The model under review builds one solid part; all positions refer to its coordinate system, in mm. A direction names the side the tool comes from. Coordinates: 2 decimals unless noted, no trailing zeros. Loops run counter-clockwise (first coordinate to the right, second up) from the corner with the lowest first, then second, coordinate; pieces in that order, holes last. Notation, with made-up numbers: M -19.5,45.5 L 16.5,45.5 A16 ccw 16.5,74.5 Z; hole C 14.25,42.5 d7. An arc over 180 degrees is marked long. One line per item, written item: value.
```python
from build123d import *

# Parameters (mm, degrees)
F0_W          = 41.3257516921
F0_H          = 115.0570958853
F1_DEPTH      = 8
F3_DEPTH      = 16
F5_DEPTH      = 8.5
F6_R          = 4
F7_R          = 10
F9_D          = 5
F10_R         = 1
F12_DEPTH     = 8
F13_T4_ANGLE  = 50.4345634546
F13_S5_R      = 29.5691559209
F13_T6_DEPTH  = 16
F13_T11_ANGLE = 49.9258142249
F13_S12_R     = 29.5691559209
F13_T13_DEPTH = 16
F14_W         = 7.5
F14_H         = 18
F15_DEPTH     = 3
F16_R         = 1


# Not quite as in the source:
# - a fillet or chamfer that OpenCascade refuses, or shapes differently, is made with other operations: its cross-section is extruded or revolved along the edge and cut away or added
# - a pattern or mirror of a feature is missing from the dataset's text; its kind, count and spacing are read off the source's solid


with BuildPart() as f1:
    # F0 (on Front) → F1 (new body)
    with BuildSketch(Plane.XZ):
        Rectangle(F0_W, F0_H)
    extrude(amount=F1_DEPTH)

    # F2 (on face) → F3 (join)
    with BuildSketch(Plane.XZ):
        with BuildLine():
            Line((20.662875846, -21.1513721457), (20.662875846, 21.1513721457))
            ThreePointArc((20.662875846, 21.1513721457), (0, 29.5691559209), (-20.662875846, 21.1513721457))
            Line((-20.662875846, 21.1513721457), (-20.662875846, -21.1513721457))
            ThreePointArc((-20.662875846, -21.1513721457), (0, -29.5691559209), (20.662875846, -21.1513721457))
        make_face()
        with BuildLine():
            ThreePointArc((20.662875846, -21.1513721457), (27.251777736, -11.4749985666), (29.5691559209, 0))
            ThreePointArc((29.5691559209, 0), (27.251777736, 11.4749985666), (20.662875846, 21.1513721457))
            Line((20.662875846, 21.1513721457), (20.662875846, -21.1513721457))
        make_face()
    extrude(amount=F3_DEPTH)

    # F4 (on face) → F5 (cut)
    with BuildSketch(Plane(origin=(0, 0, 0), x_dir=(-1, 0, 0), z_dir=(0, 1, 0))):
        Polygon((5.0357980654, 39.4895523787), (5.0357980654, 47.5048683584), (-5.0371875986, 47.5048683584), (-5.0371875986, 39.4847430289), align=None)
    f5 = extrude(amount=-F5_DEPTH, mode=Mode.SUBTRACT)

    # F5_copies: F5 across plane
    add(f5.mirror(Plane(origin=(0, 0, 0), x_dir=(-1, 0, 0), z_dir=(0, 0, -1))), mode=Mode.SUBTRACT)

    # F6
    f6_edges = [f1.edges().sort_by_distance(p)[0] for p in [
        (5.037188, -4, -47.504868),
        (-5.035798, -4, -47.504868),
        (5.037188, -4, -39.484743),
        (-5.035798, -4, -39.489552),
        (-5.035798, -4, 47.504868),
        (-5.035798, -4, 39.489552),
        (5.037188, -4, 39.484743),
        (5.037188, -4, 47.504868),
    ]]
    fillet(f6_edges, radius=F6_R)

    # F7
    f7_edges = [f1.edges().sort_by_distance(p)[0] for p in [
        (20.662876, -4, 57.528548),
        (-20.662876, -4, 57.528548),
        (-20.662876, -4, -57.528548),
        (20.662876, -4, -57.528548),
    ]]
    fillet(f7_edges, radius=F7_R)

    # F8: union 

    # F9 (through all)
    with Locations(Plane(origin=(0, 0, 0), x_dir=(1, 0, 0), z_dir=(0, 1, 0))):
        with Locations((22.990738973, 0), (-11.4866392687, -19.9111644179), (-11.4866392687, 19.9130717665)):
            Hole(F9_D / 2)

    # F10
    f10_edges = [f1.edges().sort_by_distance(p)[0] for p in [
        (-20.662876, -8, 34.33996),
        (-20.662876, -8, -34.33996),
    ]]
    fillet(f10_edges, radius=F10_R)

    # F11 (on face) → F12 (join)
    with BuildSketch(Plane.XZ.offset(16)):
        with BuildLine():
            ThreePointArc((-20.662875846, 21.1513721457), (-27.2355425635, 11.47094423), (-29.5438040048, 0))
            ThreePointArc((-29.5438040048, 0), (-27.2133537023, -11.4616276864), (-20.662875846, -21.1513721457))
            Line((-20.662875846, -21.1513721457), (-20.662875846, 21.1513721457))
        make_face()
    extrude(amount=-F12_DEPTH)

    # F13: fillet of radius 1 on 2 edges, made by hand


with BuildPart() as f13_tool2:
    # F13_s3 → F13_t4 (revolve)
    with BuildSketch(Plane(origin=(0.039948819, 0, 0.0330329638), x_dir=(0, 1, 0), z_dir=(0.7706607763, 0, 0.6372456103))):
        with BuildLine():
            ThreePointArc((-9, 29.573386115), (-8.2928932188, 29.2804928962), (-8, 28.573386115))
            Line((-8, 28.573386115), (-7.98, 28.573386115))
            Line((-7.98, 28.573386115), (-7.98, 29.593386115))
            Line((-7.98, 29.593386115), (-9, 29.593386115))
            Line((-9, 29.593386115), (-9, 29.573386115))
        make_face()
    revolve(axis=Axis((0.058163466, -8, 0.0110048576), (0, -1, 0)), revolution_arc=F13_T4_ANGLE)

    # F13_s5 → F13_t6 (intersect, symmetric)
    with BuildSketch(Plane.XZ.offset(8.5)):
        Circle(F13_S5_R)
    extrude(amount=F13_T6_DEPTH, both=True, mode=Mode.INTERSECT)

    split(bisect_by=Plane.YZ.offset(-20.662875846), keep=Keep.BOTTOM)


with BuildPart() as f1_1:
    add(f1.part)

    # F13_t1: cut F13_tool2
    add(f13_tool2.part, mode=Mode.SUBTRACT)


with BuildPart() as f13_tool9:
    # F13_s10 → F13_t11 (revolve)
    with BuildSketch(Plane(origin=(-0.0003962248, 0, 0.1081934909), x_dir=(0, 1, 0), z_dir=(-0.0036621627, 0, 0.9999932943))):
        with BuildLine():
            ThreePointArc((-9, 29.5436058917), (-8.2928932188, 29.2507126729), (-8, 28.5436058917))
            Line((-8, 28.5436058917), (-7.98, 28.5436058917))
            Line((-7.98, 28.5436058917), (-7.98, 29.5636058917))
            Line((-7.98, 29.5636058917), (-9, 29.5636058917))
            Line((-9, 29.5636058917), (-9, 29.5436058917))
        make_face()
    revolve(axis=Axis((0.3450668448, -8, 0.1094586414), (0, -1, 0)), revolution_arc=F13_T11_ANGLE)

    # F13_s12 → F13_t13 (intersect, symmetric)
    with BuildSketch(Plane.XZ.offset(8.5)):
        Circle(F13_S12_R)
    extrude(amount=F13_T13_DEPTH, both=True, mode=Mode.INTERSECT)

    split(bisect_by=Plane.YZ.offset(-20.662875846), keep=Keep.BOTTOM)


with BuildPart() as f1_2:
    add(f1_1.part)

    # F13_t8: cut F13_tool9
    add(f13_tool9.part, mode=Mode.SUBTRACT)

    # F14 (on face) → F15 (join)
    with BuildSketch(Plane(origin=(0, 0, 0), x_dir=(-1, 0, 0), z_dir=(0, 1, 0))):
        with Locations((0, -21)):
            Rectangle(F14_W, F14_H)
        with Locations((0, 21)):
            Rectangle(F14_W, F14_H)
    extrude(amount=F15_DEPTH)

    # F16
    f16_edges = [f1_2.edges().sort_by_distance(p)[0] for p in [
        (3.75, 3, 21),
        (0, 3, 12),
        (-3.75, 3, 21),
        (0, 3, 30),
        (0, 3, -12),
        (3.75, 3, -21),
        (0, 3, -30),
        (-3.75, 3, -21),
    ]]
    fillet(f16_edges, radius=F16_R)


solid = f1_2.part
```
(1) To check wall thickness, follow L1, parallel to Z at x = 3.5, y = -7.5; L2, parallel to X at y = -4.75, z = -33; L3, parallel to Y at x = 15, z = -26.5. State the ranges of each line that lie inside material, in increasing order. Write a range as [from, to].
Checks:
L1: [-57.39, -46.66], [-40.33, 40.33], [46.66, 57.39]
L2: [-20.66, 20.66]
L3: [-8, 0]
(2) Insertion check: pin 1 Ø4 at (x, z) = (21.5, 37) entering from -Y; pin 2 Ø8.5 at (x, z) = (-25, 7) entering from +Y; pin 3 Ø6 at (x, z) = (-23.5, -28) entering from +Y. Each pin has a flat end and moves straight along its axis. Give the tip position at first contact, or say it passes through.
Checks:
pin 1: y = -8
pin 2: y = -8
pin 3: y = 0
(3) Draft analysis for pull direction Z (two halves, no side actions). For faces 1 (the face through (17.656, -3.549, 54.677)), 2 (the face through (20.7, -8.1, 1)), 3 (the face through (20.663, -3, 34)), state which applies: pulls with the +Z half, pulls with the -Z half, needs draft (parallel to the pull), parting line crosses it, or undercut.
Checks:
face 1: pulls with the +Z half
face 2: undercut
face 3: needs draft
(4) Tool access review of faces 4 (the face through (-3.895, -4.056, 46.302)), 5 (the face through (-24, -8, 0)), 6 (the face through (0, 1, -30)), 7 (the face through (0, 1, -12)): name each direction out of +Z, -Z, +X, -X, +Y, -Y from which nothing blocks a thin tool from reaching the whole face with its end or side.
Checks:
face 4: +Y, -Y
face 5: +Z, -Z, -X, +Y
face 6: -Z, +X, -X, +Y
face 7: +X, -X, +Y
(5) Add section D-D on y = -1.75. State how many separate pieces and enclosed holes the cut face has, then the cut area to 3 significant figures.
Checks:
separate pieces: 1
enclosed holes: 5
area: 4,740 mm^2
(6) Add section C-C on y = -12. State the section outline as (x, z) points.
Checks:
outline: M -29.54,0 A29.89 ccw -20.66,-21.15 A29.57 ccw long -20.66,21.15 A29.6 ccw Z; hole C -11.49,-19.91 d5; hole C -11.49,19.91 d5; hole C 22.99,0 d5
(7) Add section A-A on z = 38. State the section outline as (x, y) points.
Checks:
outline: M -20.66,-7 A1 ccw -19.66,-8 L 19.66,-8 A1 ccw 20.66,-7 L 20.66,0 L -20.66,0 Z
(8) Add section B-B on z = -46. State the section outline as (x, y) points.
Checks:
outline: M -20.66,-7 A1 ccw -19.66,-8 L -4.16,-8 L -4.16,0 L -20.66,0 Z; M 4.16,-8 L 19.66,-8 A1 ccw 20.66,-7 L 20.66,0 L 4.16,0 Z
